Read the model definition and answer for the solid it produces. Units are mm, in the model's axes. A direction names the side the tool comes from. Coordinates: 2 decimals unless noted, no trailing zeros. Order: outer loops, then holes, each group sorted by start corner. A loop starts at its lowest first (then second) coordinate and runs counter-clockwise, first axis right, second up.
```python
from build123d import *

# Parameters (mm, degrees)
SKETCH_1_W          = 17.8
SKETCH_1_H          = 2.7
EXTRUDE_1_DEPTH     = 4.6
SKETCH_2_R          = 6
EXTRUDE_2_DEPTH     = 19
EXTRUDE_3_DEPTH     = 1.6
BOSS_EXTRUDE2_DEPTH = 3
SKETCH_6_R          = 3.6
CUT_EXTRUDE2_DEPTH  = 24.544850817


with BuildPart() as part:
    # 草图1 → 凸台-拉伸1 (new body)
    with BuildSketch(Plane(origin=(0, 0, 0), x_dir=(1, 0, 0), z_dir=(0, 1, 0))):
        Rectangle(SKETCH_1_W, SKETCH_1_H)
    extrude(amount=EXTRUDE_1_DEPTH)

    # 草图2 → 凸台-拉伸2 (add)
    with BuildSketch(Plane(origin=(0, 0, 0), x_dir=(-1, 0, 0), z_dir=(0, -1, 0))):
        with Locations(Location((0, 0, 0), (0, 0, 90))):
            Circle(SKETCH_2_R)
    extrude(amount=-EXTRUDE_2_DEPTH)

    # 草图4 → 凸台-拉伸3 (add)
    with BuildSketch(Plane(origin=(0, 19, 0), x_dir=(1, 0, 0), z_dir=(0, 1, 0))):
        Polygon((-5.747717471, 1.077984288), (-3.323048318, -1.346684865), (1.346684865, 3.323048318), (-1.077984288, 5.747717471), align=None)
        Polygon((-1.346684865, -3.323048318), (1.077984288, -5.747717471), (5.747717471, -1.077984288), (3.323048318, 1.346684865), align=None)
    extrude(amount=EXTRUDE_3_DEPTH)

    # Sketch4 → Boss-Extrude2 (add)
    with BuildSketch(Plane(origin=(0, 7.4, 0), x_dir=(1, 0, 0), z_dir=(0, 1, 0))):
        with BuildLine():
            ThreePointArc((6.708203932, 2), (0, 7), (-6.708203932, 2))
            Line((-6.708203932, 2), (6.708203932, 2))
        make_face()
        with BuildLine():
            ThreePointArc((-6.708203932, 2), (-6.926666858, 1.010587075), (-7, 0))
            Line((-7, 0), (7, 0))
            ThreePointArc((7, 0), (6.926666858, 1.010587075), (6.708203932, 2))
            Line((6.708203932, 2), (-6.708203932, 2))
        make_face()
        with BuildLine():
            ThreePointArc((-6.708203932, -2), (-6.926666858, -1.010587075), (-7, 0))
            ThreePointArc((-7, 0), (-6.926666858, 1.010587075), (-6.708203932, 2))
            Line((-6.708203932, 2), (-7, 2))
            ThreePointArc((-7, 2), (-9, 0), (-7, -2))
            Line((-7, -2), (-6.708203932, -2))
        make_face()
        with BuildLine():
            Line((7, 0), (-7, 0))
            ThreePointArc((-7, 0), (-6.926666858, -1.010587075), (-6.708203932, -2))
            Line((-6.708203932, -2), (6.708203932, -2))
            ThreePointArc((6.708203932, -2), (6.926666858, -1.010587075), (7, 0))
        make_face()
        with BuildLine():
            Line((6.708203932, -2), (-6.708203932, -2))
            ThreePointArc((-6.708203932, -2), (0, -7), (6.708203932, -2))
        make_face()
        with BuildLine():
            ThreePointArc((6.708203932, 2), (6.926666858, 1.010587075), (7, 0))
            ThreePointArc((7, 0), (6.926666858, -1.010587075), (6.708203932, -2))
            Line((6.708203932, -2), (7, -2))
            ThreePointArc((7, -2), (9, 0), (7, 2))
            Line((7, 2), (6.708203932, 2))
        make_face()
    extrude(amount=BOSS_EXTRUDE2_DEPTH)

    # 草图6 → Cut-Extrude2 (cut, through all)
    with BuildSketch(Plane.XZ):
        with Locations(Location((0, 0, 0), (0, 0, 270))):
            Circle(SKETCH_6_R)
    extrude(amount=-CUT_EXTRUDE2_DEPTH, mode=Mode.SUBTRACT)


solid = part.part
```
1) A cutting plane is placed at B-B, the plane x = 7.25. Determine the outline of the cut face in (y, z).
A:
outline: (0, -1.35) - (4.6, -1.35) - (4.6, 1.35) - (0, 1.35) - close; (7.4, -1.98) - (10.4, -1.98) - (10.4, 1.98) - (7.4, 1.98) - close
2) Determine the mould class of faces 1 (the flat face through (4.57, 19.79, -0.1)), 2 (the cylindrical face through (-3.194, 10.156, -1.661)), 3 (the flat face through (-7, 2, -1.35)) for opening direction X: pulls with the +X half, pulls with the -X half, needs draft (parallel to the pull), parting line crosses it, or undercut.
A:
face 1: pulls with the +X half
face 2: undercut
face 3: needs draft
3) A cutting plane is placed at D-D, the plane x = -0.5. Determine the outline of the cut face in (y, z).
A:
outline: (0, -5.98) - (7.4, -5.98) - (7.4, -6.98) - (10.4, -6.98) - (10.4, -5.98) - (19, -5.98) - (19, -5.17) - (20.6, -5.17) - (20.6, -3.57) - (0, -3.57) - close; (0, 3.57) - (20.6, 3.57) - (20.6, 4.17) - (19, 4.17) - (19, 5.98) - (10.4, 5.98) - (10.4, 6.98) - (7.4, 6.98) - (7.4, 5.98) - (0, 5.98) - close
4) A cutting plane is placed at C-C, the plane z = 0. Determine the outline of the cut face in (x, y).
A:
outline: (-9, 7.4) - (-6, 7.4) - (-6, 4.6) - (-8.9, 4.6) - (-8.9, 0) - (-3.6, 0) - (-3.6, 20.6) - (-4.67, 20.6) - (-4.67, 19) - (-6, 19) - (-6, 10.4) - (-9, 10.4) - close; (3.6, 0) - (8.9, 0) - (8.9, 4.6) - (6, 4.6) - (6, 7.4) - (9, 7.4) - (9, 10.4) - (6, 10.4) - (6, 19) - (4.67, 19) - (4.67, 20.6) - (3.6, 20.6) - close
5) Which of the six approach directions +Z, -Z, +X, -X, +Y, -Y give full straight-line access (tool end or side, diameter ignored) to faces 4 (the flat face through (2, 7.4, -6)), 5 (the flat face through (3, 19, -3)), 6 (the flat face through (-8.9, 2, 0))?
A:
face 4: none
face 5: +Y
face 6: +Z, -Z, -X, -Y
6) Flat-ended cylindrical pins translate along their axes: pin 1 Ø1.5 at (x, y) = (-8, 2) entering from -Z; pin 2 Ø0.9 at (x, y) = (7.5, 1.5) entering from +Z; pin 3 Ø0.8 at (x, z) = (6.5, 0) entering from +Y. Find the tip coordinate at first contact, or state that the pin passes through.
A:
pin 1: stops at z = -1.35
pin 2: stops at z = 1.35
pin 3: stops at y = 10.4
7) A cutting plane is placed at A-A, the plane y = 9.75. Determine the outline of the cut face in (x, z).
A:
outline: (-7, -2) - (-6.71, -2) arc R7 ccw to (6.71, -2) - (7, -2) arc R2 ccw to (7, 2) - (6.71, 2) arc R7 ccw to (-6.71, 2) - (-7, 2) arc R2 ccw to start; hole circle Ø7.2 at (0, 0)
8) Straight lines are drawn through the part: line 1 (X direction, y = 14.5, z = 0); line 2 (X direction, y = 10.25, z = 0); line 3 (Y direction, x = 2.75, z = 5). For each, find the intervals that lie inside material, in ascending order.
A:
line 1: x = -6 to -3.6, 3.6 to 6
line 2: x = -9 to -3.6, 3.6 to 9
line 3: y = 0 to 19
